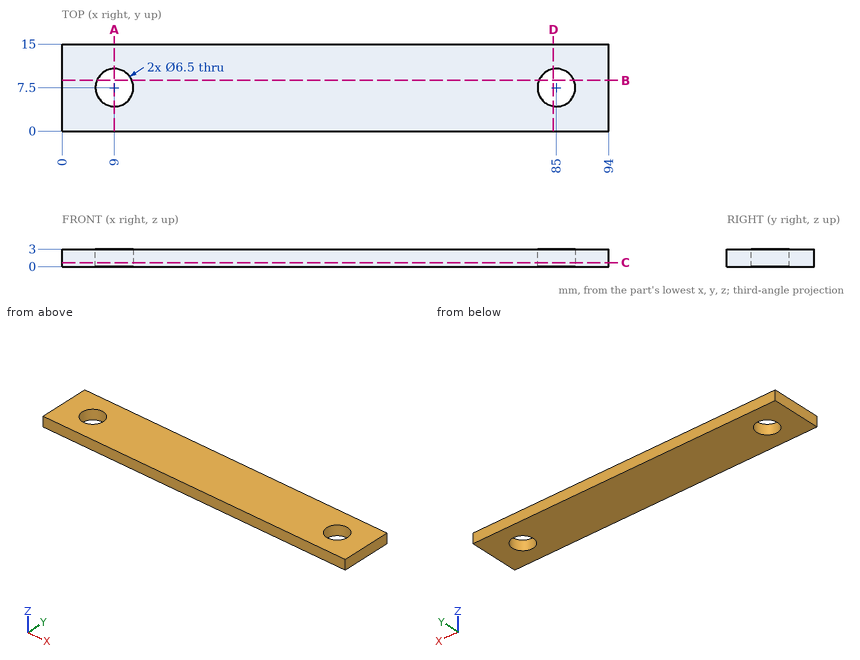
Check sheet for the drawn part. Datum: minimum x, y, z corner. Units: mm. Round coordinates to 2 decimals unless told otherwise and drop trailing zeros. Order: outer loops, then holes, each group sorted by start corner. A loop starts at its lowest first (then second) coordinate and runs counter-clockwise, first axis right, second up. Notation, with made-up numbers: (-34.5, 87.5) - (-29.5, 87.5) arc R15 cw to (-29.5, 91.5) - close; hole circle Ø4 at (42, 44.25). An arc over 180 degrees is marked (long way). Use a Markdown table: item, result. Add a question column.
(1) Material ranges on line 1 along X through (y, z) = (7.25, 1.2); line 2 along X through (y, z) = (8.5, 1.3); line 3 along Y through (x, z) = (85, 2.2), recorded low to high. Write a range as [from, to].
(2) Sectioned sample at B-B, the plane y = 8.75. Enter the section's corners in (x, z), and give its area (3 significant figures).
(3) Sectioned sample at D-D, the plane x = 84.5. Enter the section's corners in (y, z), and give its area (3 significant figures).
(4) Sectioned sample at A-A, the plane x = 9. Enter the section's corners in (y, z).
(5) Depth check by flat-ended pin: pin 1 (6 mm diameter, centred on x = 9, y = 7.5, fed in from +Z). Enter the tip coordinate at first touch or a pass-through.
(6) Sectioned sample at C-C, the plane z = 0.7. Enter the section's corners in (x, y), and give its area (3 significant figures).
Answers below:
| question | item | result |
|---|---|---|
| 1 | line 1 | [0, 5.76], [12.24, 81.76], [88.24, 94] |
| 1 | line 2 | [0, 5.91], [12.09, 81.91], [88.09, 94] |
| 1 | line 3 | [0, 4.25], [10.75, 15] |
| 2 | outline | (0, 0) - (6, 0) - (6, 3) - (0, 3) - close; (12, 0) - (82, 0) - (82, 3) - (12, 3) - close; (88, 0) - (94, 0) - (94, 3) - (88, 3) - close |
| 2 | area | 246 mm² |
| 3 | outline | (0, 0) - (4.29, 0) - (4.29, 3) - (0, 3) - close; (10.71, 0) - (15, 0) - (15, 3) - (10.71, 3) - close |
| 3 | area | 25.7 mm² |
| 4 | outline | (0, 0) - (4.25, 0) - (4.25, 3) - (0, 3) - close; (10.75, 0) - (15, 0) - (15, 3) - (10.75, 3) - close |
| 5 | pin 1 | through |
| 6 | outline | (0, 0) - (94, 0) - (94, 15) - (0, 15) - close; hole circle Ø6.5 at (9, 7.5); hole circle Ø6.5 at (85, 7.5) |
| 6 | area | 1,340 mm² |
